```python
from build123d import *

# Parameters (mm, degrees)
F1_DEPTH  = 12.7
F4_DEPTH  = 3.81
F6_DEPTH  = 8.636
F8_DEPTH  = 29.211
F9_R      = 2.667
F10_DEPTH = 4.318
F12_DEPTH = 5.08
F13_R     = 1.27
F14_DEPTH = 12.7
F15_R     = 5.715
F16_DEPTH = 2.794
F17_W     = 29.21
F17_H     = 12.7
F18_DEPTH = 11.43
F19_R     = 0.2


with BuildPart() as f1:
    # F0 (on Front) → F1 (new body)
    with BuildSketch(Plane.XZ):
        Polygon((-14.605, -3.7465), (14.605, -3.7465), (14.605, 3.7465), (14.605, 18.3515), (-14.605, 18.3515), (-14.605, 3.7465), align=None)
    extrude(amount=F1_DEPTH)

    # F3 (on offset) → F4 (cut)
    with BuildSketch(Plane.XZ.offset(6.35)):
        with BuildLine():
            Line((-9.144, -3.7465), (9.144, -3.7465))
            Line((9.144, -3.7465), (9.144, 6.9215))
            ThreePointArc((9.144, 6.9215), (0, 16.0655), (-9.144, 6.9215))
            Line((-9.144, 6.9215), (-9.144, -3.7465))
        make_face()
    extrude(amount=F4_DEPTH, mode=Mode.SUBTRACT)

    # F5 (on face) → F6 (cut)
    with BuildSketch(Plane.XZ.offset(12.7)):
        with BuildLine():
            Line((6.35, -3.7465), (4.8460111432, 5.3975))
            ThreePointArc((4.8460111432, 5.3975), (0, 12.0015), (-4.8460111432, 5.3975))
            Line((-4.8460111432, 5.3975), (-6.35, -3.7465))
            Line((-6.35, -3.7465), (6.35, -3.7465))
        make_face()
    extrude(amount=-F6_DEPTH, mode=Mode.SUBTRACT)

    # F7 (on face) → F8 (cut, through all)
    with BuildSketch(Plane.YZ.offset(14.605)):
        Polygon((-2.032, -0.6985), (0, -1.7145), (0, 16.3195), (-2.032, 15.3035), align=None)
    extrude(amount=-F8_DEPTH, mode=Mode.SUBTRACT)

    # F9 (on face) → F10 (cut, through all)
    with BuildSketch(Plane(origin=(0, -2.032, 0), x_dir=(-1, 0, 0), z_dir=(0, 1, 0))):
        with Locations((0, 6.9215)):
            Circle(F9_R)
    extrude(amount=-F10_DEPTH, mode=Mode.SUBTRACT)

    # F11 (on face) → F12 (cut)
    with BuildSketch(Plane.XY.offset(18.3515)):
        with BuildLine():
            Line((14.605, -4.191), (11.43, -4.191))
            ThreePointArc((11.43, -4.191), (8.255, -7.366), (11.43, -10.541))
            Line((11.43, -10.541), (14.605, -10.541))
            Line((14.605, -10.541), (14.605, -4.191))
        make_face()
        with BuildLine():
            ThreePointArc((-11.43, -10.541), (-8.255, -7.366), (-11.43, -4.191))
            Line((-11.43, -4.191), (-14.605, -4.191))
            Line((-14.605, -4.191), (-14.605, -10.541))
            Line((-14.605, -10.541), (-11.43, -10.541))
        make_face()
    extrude(amount=-F12_DEPTH, mode=Mode.SUBTRACT)

    # F13 (on face) → F14 (cut)
    with BuildSketch(Plane.XY.offset(13.2715)):
        with Locations((11.43, -7.366)):
            Circle(F13_R)
        with Locations((-11.43, -7.366)):
            Circle(F13_R)
    extrude(amount=-F14_DEPTH, mode=Mode.SUBTRACT)

    # F15 (on face) → F16 (cut)
    with BuildSketch(Plane.XZ.offset(6.35)):
        with Locations((0, 6.9215)):
            Circle(F15_R)
    extrude(amount=-F16_DEPTH, mode=Mode.SUBTRACT)

    # F17 (on face) → F18 (cut)
    with BuildSketch(Plane.XY.offset(18.3515)):
        with Locations((0, -6.35)):
            Rectangle(F17_W, F17_H)
    extrude(amount=-F18_DEPTH, mode=Mode.SUBTRACT)

    # F19
    f19_edges = [f1.edges().sort_by_distance(p)[0] for p in [
        (14.605, -12.7, 1.5875),
        (5.021162, -12.7, 6.150571),
        (5.598006, -12.7, 0.8255),
        (5.021162, -10.16, 6.150571),
        (5.598006, -10.16, 0.8255),
        (5.543389, -6.35, 5.531512),
        (5.694431, -6.35, 0.239251),
        (-5.021162, -12.7, 6.150571),
        (-5.021162, -10.16, 6.150571),
        (-5.598006, -10.16, 0.8255),
        (-5.598006, -12.7, 0.8255),
        (-5.543389, -6.35, 5.531512),
        (-5.694431, -6.35, 0.239251),
        (0, -4.064, 1.2065),
        (0, -3.556, 4.2545),
        (0, -2.032, 4.2545),
        (14.605, -2.032, 3.1115),
        (-14.605, -2.032, 3.1115),
        (-14.605, -1.016, -1.2065),
        (-14.605, 0, -2.7305),
        (14.605, -1.016, -1.2065),
        (14.605, 0, -2.7305),
        (-14.605, -12.7, 1.5875),
    ]]
    fillet(f19_edges, radius=F19_R)


solid = f1.part
```
The listing builds one solid part. Answer for the finished solid, in the listing's coordinates (mm). A direction names the side the tool comes from. Coordinates: 2 decimals unless noted, no trailing zeros. Loops run counter-clockwise (first coordinate to the right, second up) from the corner with the lowest first, then second, coordinate; pieces in that order, holes last. Notation, with made-up numbers: (-8.5, 37.25) - (36.5, 37.25) arc R36 cw to (36.5, 71.25) - close; hole circle Ø7 at (-18, 60). An arc over 180 degrees is marked (long way). Use a Markdown table: item, result. Add a question column.
1) The part is cut by section B-B, the plane x = -11.43. Give the vertices of the cut face in (y, z), and give its area (3 significant figures).
2) Find the intervals of material crossed by line 1 (Y direction, x = -11.43, z = 4.75); line 2 (Y direction, x = -6.75, z = 1); line 3 (X direction, y = -6.75, z = -2.5) (3 decimals), in increasing order.
3) For faces 5 (the cylindrical face through (5.646, -10.22, 0.883)), 6 (the cylindrical face through (-5.023, -11.445, 6.161)), 7 (the flat face through (-8, -10.16, 2)), 8 (the flat face through (11, -7, 0.572)), 9 (the flat face through (-5.587, -11.445, 0.89)), determine the directions among +Z, -Z, +X, -X, +Y, -Y from which every point of the face is accessible in a straight line to the end or side of a thin tool.
4) Given pin 1 (4 mm diameter, centred on x = -7.5, z = 5.5, fed in from +Y); pin 2 (6 mm diameter, centred on x = -2, z = -1, fed in from -Y); pin 3 (0.8 mm diameter, centred on x = 11, y = -7, fed in from +Z), each flat-ended and moving along its own axis, determine where each tip first touches the part or whether it passes through.
5) The mould has two halves that part along X. Classify faces 1 (the cylindrical face through (-5.67, -12.64, 0.75)), 2 (the flat face through (0, -2.032, 3)), 3 (the flat face through (-14.605, -8, 2)), 4 (the cylindrical face through (5.649, -12.643, 0.883)): released by +X, released by -X, zero draft, split by the parting line, or undercut.
6) The part is cut by section D-D, the plane z = 1.5. State how many separate pieces and enclosed holes the cut face has, and give its area (3 significant figures).
7) The part is cut by section C-C, the plane x = 0. Give the vertices of the cut face in (y, z), and give its area (3 significant figures).
Here are the results:
| question | item | result |
|---|---|---|
| 1 | outline | (-12.7, -3.75) - (0, -3.75) - (0, -1.71) - (-2.03, -0.7) - (-2.03, 6.92) - (-6.1, 6.92) - (-6.1, 0.57) - (-8.64, 0.57) - (-8.64, 6.92) - (-12.7, 6.92) - close |
| 1 | area | 103 mm^2 |
| 2 | line 1 | y = -12.7 to -8.64, -6.1 to -2.03 |
| 2 | line 2 | y = -12.7 to -10.16, -6.35 to -2.03 |
| 2 | line 3 | x = -14.605 to -9.144, 9.144 to 14.605 |
| 3 | face 5 | -Z |
| 3 | face 6 | +Z, -Y |
| 3 | face 7 | +Z, -Z |
| 3 | face 8 | +Z |
| 3 | face 9 | -Z, -Y |
| 4 | pin 1 | stops at y = -2.03 |
| 4 | pin 2 | stops at y = -4.06 |
| 4 | pin 3 | stops at z = 0.57 |
| 5 | face 1 | undercut |
| 5 | face 2 | zero draft |
| 5 | face 3 | released by -X |
| 5 | face 4 | undercut |
| 6 | separate pieces | 1 |
| 6 | enclosed holes | 2 |
| 6 | area | 177 mm^2 |
| 7 | outline | (-4.06, -3.75) - (0, -3.75) - (0, -1.71) - (-2.03, -0.7) - (-2.03, 4.05) arc R0.2 ccw to (-2.23, 4.25) - (-3.36, 4.25) arc R0.2 ccw to (-3.56, 4.05) - (-3.56, 1.21) - (-3.86, 1.21) arc R0.2 ccw to (-4.06, 1.01) - close |
| 7 | area | 19.8 mm^2 |
